For this review, take the finished solid that the model builds, in its own axes (mm). Face numbers are marked on the shaded views. A direction names the side the tool comes from. Give positions to 0.01 mm unless a question says otherwise; leave off trailing zeros. Order: outer loops, then holes, each group sorted by start corner. A loop starts at its lowest first (then second) coordinate and runs counter-clockwise, first axis right, second up. Notation, with made-up numbers: (55, 0.25) -> (100, 0.25) arc R10 ccw to (100, 8.25) -> close; hole circle Ø4 at (9.5, 61). An arc over 180 degrees is marked (long way). Return JSON: item names as keys, results as strings. Group by question number.
1) To check wall thickness, follow line 1 along X through (y, z) = (8.5, 1); line 2 along Y through (x, z) = (76.5, -8); line 3 along X through (y, z) = (9.25, 78). State the ranges of each line that lie inside material, in increasing order.
2) Insertion check: P1, Ø2.5, axis at x = -62.5, y = 26.5, coming from the -Z side; P2, Ø5, axis at x = -85.5, z = 3, coming from the +Y side; P3, Ø8, axis at y = 11.5, z = 20.5, coming from the -X side. Each pin has a flat end and moves straight along its axis. Give the tip position at first contact, or say it passes through.
3) For the marked faces 4 and 5, list the 3-axis set-ups (+Z, -Z, +X, -X, +Y, -Y) from which the entire face can be reached by the end or side of a thin tool; tool diameter is ignored.
4) Add section C-C (z = -41). Give the boundary of the cut face in (x, y) (3 decimals), then the cut area to 3 significant figures.
5) The part is to be moulded in two halves that separate along Y. For the marked faces 1, 2 and 3, say which applies: released by +Y, released by -Y, zero draft, split by the parting line, or undercut.
6) Add section B-B (x = 0). Give the boundary of the cut face in (y, z) (3 decimals), then the cut area to 3 significant figures.
7) Add section A-A (y = 20.75). Give the boundary of the cut face in (x, z) (3 decimals), then the cut area to 3 significant figures.
8) Add section D-D (y = 3.75). Give the boundary of the cut face in (x, z) (3 decimals).
from build123d import *

# Parameters (mm, degrees)
SKETCH1_R                = 63.5
SKETCH1_R_2              = 55.88
BOSS_EXTRUDE1_DEPTH      = 9.525
BOSS_EXTRUDE2_DEPTH      = 15.875
BOSS_EXTRUDE2_DEPTH_BACK = 9.525
BOSS_EXTRUDE3_DEPTH      = 3.175
CIRPATTERN1_COUNT        = 6
BOSS_EXTRUDE7_DEPTH      = 9.525
CUT_EXTRUDE5_DEPTH       = 6.35
CUT_EXTRUDE8_START       = -15.875
CUT_EXTRUDE8_DEPTH       = 15.875
CUT_EXTRUDE10_DEPTH      = 10.414


with BuildPart() as part:
    # Sketch1 → Boss-Extrude1 (new body)
    with BuildSketch(Plane(origin=(0, 0, 0), x_dir=(1, 0, 0), z_dir=(0, 1, 0))):
        with Locations(Location((0, 0, 0), (0, 0, 90))):
            Circle(SKETCH1_R)
        with Locations(Location((0, 0, 0), (0, 0, 90))):
            Circle(SKETCH1_R_2, mode=Mode.SUBTRACT)
    extrude(amount=BOSS_EXTRUDE1_DEPTH)

    # Sketch2 → Boss-Extrude2 (add, two sides: drawn at the far end of the back side and taken through both)
    with BuildSketch(Plane(origin=(0, 9.525, 0), x_dir=(1, 0, 0), z_dir=(0, 1, 0)).offset(-BOSS_EXTRUDE2_DEPTH_BACK)):
        with BuildLine():
            ThreePointArc((62.042091837, 13.528815193), (75.175517225, 12.909752551), (86.858928571, 18.94034127))
            ThreePointArc((86.858928571, 18.94034127), (97.349634921, 10.490706349), (88.9, 0))
            ThreePointArc((88.9, 0), (76.2, 3.402954744), (63.5, 0))
            ThreePointArc((63.5, 0), (63.1344709, 6.803571429), (62.042091837, 13.528815193))
        make_face()
    extrude(amount=BOSS_EXTRUDE2_DEPTH + BOSS_EXTRUDE2_DEPTH_BACK)

    # Sketch3 → Boss-Extrude3 (add)
    with BuildSketch(Plane(origin=(0, 25.4, 0), x_dir=(1, 0, 0), z_dir=(0, 1, 0))):
        with BuildLine():
            Line((60.325, 0), (63.5, 0))
            ThreePointArc((63.5, 0), (65.659371798, 1.11258817), (67.915149907, 2.013811849))
            ThreePointArc((67.915149907, 2.013811849), (67.553883863, 7.279821429), (66.784920566, 12.501896255))
            ThreePointArc((66.784920566, 12.501896255), (64.388925587, 12.901830068), (62.042091837, 13.528815193))
            Line((62.042091837, 13.528815193), (58.939987245, 12.852374433))
            ThreePointArc((58.939987245, 12.852374433), (59.977747355, 6.463392857), (60.325, 0))
        make_face()
    extrude(amount=BOSS_EXTRUDE3_DEPTH)


with BuildPart() as cirpattern1_1:
    # CirPattern1: pattern copy
    add(part.part.rotate(Axis((0, 0, 0), (0, 1, 0)), 1 * 360 / CIRPATTERN1_COUNT))


with BuildPart() as cirpattern1_2:
    # CirPattern1: pattern copy
    add(part.part.rotate(Axis((0, 0, 0), (0, 1, 0)), 2 * 360 / CIRPATTERN1_COUNT))


with BuildPart() as cirpattern1_3:
    # CirPattern1: pattern copy
    add(part.part.rotate(Axis((0, 0, 0), (0, 1, 0)), 3 * 360 / CIRPATTERN1_COUNT))


with BuildPart() as cirpattern1_4:
    # CirPattern1: pattern copy
    add(part.part.rotate(Axis((0, 0, 0), (0, 1, 0)), 4 * 360 / CIRPATTERN1_COUNT))


with BuildPart() as cirpattern1_5:
    # CirPattern1: pattern copy
    add(part.part.rotate(Axis((0, 0, 0), (0, 1, 0)), 5 * 360 / CIRPATTERN1_COUNT))


with BuildPart() as part_1:
    add(part.part)

    add(cirpattern1_1.part)  # Boss-Extrude7 merges CirPattern1_1

    add(cirpattern1_2.part)  # Boss-Extrude7 merges CirPattern1_2

    add(cirpattern1_3.part)  # Boss-Extrude7 merges CirPattern1_3

    add(cirpattern1_4.part)  # Boss-Extrude7 merges CirPattern1_4

    add(cirpattern1_5.part)  # Boss-Extrude7 merges CirPattern1_5
    # Sketch7 → Boss-Extrude7 (add)
    with BuildSketch(Plane(origin=(0, 0, 0), x_dir=(-1, 0, 0), z_dir=(0, -1, 0))):
        with BuildLine():
            Line((63.5, 0), (67.569096786, -7.577162194))
            Line((67.569096786, -7.577162194), (97.349634921, -10.490706349))
            ThreePointArc((97.349634921, -10.490706349), (97.772251641, -5.252918049), (97.91325926, 0))
            Line((97.91325926, 0), (88.9, 0))
            Line((88.9, 0), (63.5, 0))
        make_face()
    extrude(amount=-BOSS_EXTRUDE7_DEPTH)

    # Sketch9 → Cut-Extrude5 (cut)
    with BuildSketch(Plane(origin=(0, 0, 0), x_dir=(-1, 0, 0), z_dir=(0, -1, 0))):
        with BuildLine():
            Line((61.39651055, -26.00046379), (106.955649778, -39.531378336))
            Line((106.955649778, -39.531378336), (132.962005417, 11.016778764))
            Line((132.962005417, 11.016778764), (94.714323946, 43.842731985))
            Line((94.714323946, 43.842731985), (63.332617029, 20.845508994))
            ThreePointArc((63.332617029, 20.845508994), (66.618128975, -2.753273836), (61.39651055, -26.00046379))
        make_face()
    extrude(amount=-CUT_EXTRUDE5_DEPTH, mode=Mode.SUBTRACT)

    # Sketch11 → Cut-Extrude8 (cut)
    with BuildSketch(Plane(origin=(0, 25.4, 0), x_dir=(1, 0, 0), z_dir=(0, 1, 0)).offset(CUT_EXTRUDE8_START)):
        with BuildLine():
            Line((-67.842452842, -3.731570369), (-122.840055189, -6.75662938))
            Line((-122.840055189, -6.75662938), (-98.142005423, 22.287709704))
            Line((-98.142005423, 22.287709704), (-66.460403185, 14.125786119))
            ThreePointArc((-66.460403185, 14.125786119), (-67.742420826, 5.242847087), (-67.842452842, -3.731570369))
        make_face()
    extrude(amount=CUT_EXTRUDE8_DEPTH, mode=Mode.SUBTRACT)

    # Sketch12 → Cut-Extrude10 (cut)
    with BuildSketch(Plane.XZ.offset(-6.35)):
        with BuildLine():
            Line((-69.200337384, 1.380715925), (-95.001475013, 1.380715925))
            ThreePointArc((-95.001475013, 1.380715925), (-96.144492419, 2.523733331), (-95.001475013, 3.666750736))
            Line((-95.001475013, 3.666750736), (-69.200337384, 3.666750736))
            ThreePointArc((-69.200337384, 3.666750736), (-68.057319979, 2.523733331), (-69.200337384, 1.380715925))
        make_face()
    extrude(amount=-CUT_EXTRUDE10_DEPTH, mode=Mode.SUBTRACT)


solid = part_1.part
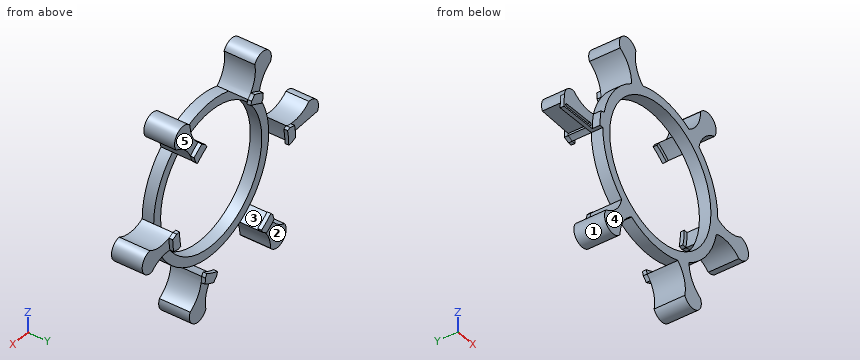
Evaluation:
{
 "1": {"line 1": "-97.91 to -55.87, 55.87 to 63.49", "line 2": "0 to 25.4", "line 3": "-44.83 to -27.58, 45.3 to 58.98"},
 "2": {"P1": "z = 0", "P2": "y = 25.4", "P3": "x = -94.31"},
 "3": {"face 4": "+Z, -Z, +X, -X, -Y", "face 5": "+Z, +X, +Y"},
 "4": {"outline": "(-48.49, 0) -> (-37.968, 0) -> (-37.968, 9.525) -> (-48.49, 9.525) -> close; (37.968, 0) -> (48.49, 0) -> (48.49, 9.525) -> (37.968, 9.525) -> close", "area": "200 mm^2"},
 "5": {"face 1": "zero draft", "face 2": "released by +Y", "face 3": "undercut"},
 "6": {"outline": "(0, -63.5) -> (9.525, -63.5) -> (9.525, -55.88) -> (0, -55.88) -> close; (0, 55.88) -> (9.525, 55.88) -> (9.525, 63.5) -> (0, 63.5) -> close", "area": "145 mm^2"},
 "7": {"outline": "(-96.445, 5.305) -> (-67.842, 3.732) arc R67.945 ccw to (-67.915, 2.014) arc R25.4 cw to (-63.5, 0) arc R63.5 cw to (-62.042, 13.529) arc R25.4 cw to (-86.859, 18.94) arc R9.525 ccw to start; (-59.832, -65.752) arc R9.525 ccw to (-44.45, -76.99) arc R25.4 cw to (-31.75, -54.993) arc R63.5 cw to (-42.737, -46.966) arc R25.4 cw to start; (-44.45, 76.99) arc R25.4 cw to (-31.75, 54.993) arc R63.5 cw to (-19.305, 60.494) arc R25.4 cw to (-27.027, 84.692) arc R9.525 ccw to start; (19.305, -60.494) arc R25.4 cw to (27.027, -84.692) arc R9.525 ccw to (44.45, -76.99) arc R25.4 cw to (31.75, -54.993) arc R63.5 cw to start; (31.75, 54.993) arc R63.5 cw to (42.737, 46.966) arc R25.4 cw to (59.832, 65.752) arc R9.525 ccw to (44.45, 76.99) arc R25.4 cw to start; (62.042, -13.529) arc R25.4 cw to (86.859, -18.94) arc R9.525 ccw to (88.9, 0) arc R25.4 cw to (63.5, 0) arc R63.5 cw to start", "area": "2,550 mm^2"},
 "8": {"outline": "(-66.675, 0) -> (-63.5, 0) arc R63.5 ccw to (-42.737, -46.966) arc R25.4 cw to (-59.832, -65.752) arc R9.525 ccw to (-44.45, -76.99) arc R25.4 cw to (-31.75, -54.993) arc R63.5 ccw to (19.305, -60.494) arc R25.4 cw to (27.027, -84.692) arc R9.525 ccw to (44.45, -76.99) arc R25.4 cw to (31.75, -54.993) arc R63.5 ccw to (62.042, -13.529) arc R25.4 cw to (86.859, -18.94) arc R9.525 ccw to (88.9, 0) arc R25.4 cw to (63.5, 0) arc R63.5 ccw to (42.737, 46.966) arc R25.4 cw to (59.832, 65.752) arc R9.525 ccw to (44.45, 76.99) arc R25.4 cw to (31.75, 54.993) arc R63.5 ccw to (-19.305, 60.494) arc R25.4 cw to (-27.027, 84.692) arc R9.525 ccw to (-44.45, 76.99) arc R25.4 cw to (-31.75, 54.993) arc R63.5 ccw to (-62.042, 13.529) arc R25.4 cw to (-65.455, 12.695) arc R66.675 ccw to start; hole circle Ø111.76 at (0, 0)"}
}
